```python
from build123d import *

# Parameters (mm, degrees)
F0_R     = 1.778
F0_W     = 19.05
F0_H     = 25.4
F0_R_2   = 1.7145
F1_DEPTH = 3.175
F2_DEPTH = 11.43


# Not quite as in the source:
# - a feature names something its author has since deleted; it is built from what else it names


with BuildPart() as f1:
    # F0 (on Top) → F1 (new body)
    with BuildSketch(Plane.XY):
        Polygon((-38.2503936946, 15.7646441165), (-38.2503936946, -9.6299967694), (139.5496063054, -9.6299967694), (139.5496063054, 15.7700032306), (12.5479004732, 15.7700032306), (-11.7069316009, 15.7700032306), (-38.2485270353, 15.7700032306), align=None)
        Polygon((20.5585099757, -3.2853558835), (20.5585099757, 3.0646441165), (20.5585099757, 9.4146441165), (25.6385099757, 9.4146441165), (25.6385099757, -3.2853558835), align=None, mode=Mode.SUBTRACT)
        Polygon((35.4481115937, -3.2853558835), (35.4481115937, 3.0646441165), (35.4481115937, 9.4146441165), (40.5281115937, 9.4146441165), (40.5281115937, -3.2853558835), align=None, mode=Mode.SUBTRACT)
        with Locations((50.6496063054, 3.0646441165)):
            Circle(F0_R, mode=Mode.SUBTRACT)
        with Locations((63.3496063054, 3.0646441165)):
            Circle(F0_R, mode=Mode.SUBTRACT)
        with Locations((76.0496063054, 3.0646441165)):
            Circle(F0_R, mode=Mode.SUBTRACT)
        with Locations((88.7496063054, 3.0646441165)):
            Circle(F0_R, mode=Mode.SUBTRACT)
        with Locations((101.4496063054, 3.0646441165)):
            Circle(F0_R, mode=Mode.SUBTRACT)
        with Locations((114.1496063054, 3.0646441165)):
            Circle(F0_R, mode=Mode.SUBTRACT)
        with Locations((126.8496063054, 3.0646441165)):
            Circle(F0_R, mode=Mode.SUBTRACT)
        Polygon((-44.6003936946, 15.7700032306), (-44.6003936946, -9.6299967694), (-38.2503936946, -9.6299967694), (-38.2503936946, 15.7646441165), (-38.2485270353, 15.7700032306), align=None)
        with Locations((-54.1253936946, 3.0700032306)):
            Rectangle(F0_W, F0_H)
        with Locations((-50.9503936946, 3.0646441165)):
            Circle(F0_R_2, mode=Mode.SUBTRACT)
        Polygon((-11.7069316009, 91.9700032306), (-38.2485270353, 15.7700032306), (-11.7069316009, 15.7700032306), align=None)
        Polygon((-11.7069316009, 91.9700032306), (-11.7069316009, 15.7700032306), (12.5479004732, 15.7700032306), align=None)
    extrude(amount=F1_DEPTH)

    # F0 (on Top) → F2 (join)
    with BuildSketch(Plane.XY):
        with Locations((-50.9503936946, 3.0646441165)):
            Circle(F0_R_2)
    extrude(amount=F2_DEPTH)


solid = f1.part
```
Could you check a few things on this model? Use its own coordinates, in mm. A direction names the side the tool comes from. Coordinates: 2 decimals unless noted, no trailing zeros. Loops run counter-clockwise (first coordinate to the right, second up) from the corner with the lowest first, then second, coordinate; pieces in that order, holes last. Notation, with made-up numbers: M 11,68.25 L 53,68.25 A28 ccw 53,105.25 Z; hole C 30.25,63 d4. An arc over 180 degrees is marked long. Put each result on its own line as item: value. Start each with the question number.
(1) Suppose I cut it at B-B on y = 13. Please give me the cut outline in (x, z) (3 decimals), then the cut area to 3 significant figures.
(2) Suppose I cut it at A-A on x = 23.5. Please give me the cut outline in (y, z) (3 decimals).
(3) Thinking about a two-plate mould opening in X: for faces 3 (the face through (115.846, 3.599, 1.565)), 4 (the face through (125.073, 3.143, 1.565)), 5 (the face through (0.6, 53.3, 1.6)), 6 (the face through (22, 11, 3.175)), which applies, pulls with the +X half, pulls with the -X half, needs draft (parallel to the pull), parting line crosses it, or undercut?
(4) Suppose I cut it at D-D on z = 8. Please give me the cut outline in (x, y), then the cut area to 3 significant figures.
(5) For faces 1 (the face through (-52.663, 3.14, 7.245)), 2 (the face through (90.446, 3.599, 1.565)), which set-ups out of +Z, -Z, +X, -X, +Y, -Y let a thin tool reach every point of the face, with its end or its side?
(6) Will these pins go through, and if not, where does the flat tip stop? P1, Ø1, axis at x = -52.5, z = 1.5, coming from the +Y side; P2, Ø5.5, axis at x = 126.85, y = 3.06, coming from the +Z side (3 decimals); P3, Ø3, axis at x = 114.15, y = 3.06, coming from the -Z side; P4, Ø3, axis at y = 75, z = 4, coming from the -X side.
(7) Suppose I cut it at C-C on x = 67.5. Please give me the cut outline in (y, z) (3 decimals).
(8) I need wall thicknesses on line 1 (Y direction, x = 24.5, z = 2.5); line 2 (Y direction, x = 72.5, z = 2.5); line 3 (Z direction, x = 84.5, y = 15) (3 decimals). Which ranges of each line are inside material? Lowest first, please. Write a range as from..to.
Solutions:
1. outline: M -63.65,0 L 139.55,0 L 139.55,3.175 L -63.65,3.175 Z
1. area: 645 mm2
2. outline: M -9.63,0 L -3.285,0 L -3.285,3.175 L -9.63,3.175 Z; M 9.415,0 L 15.77,0 L 15.77,3.175 L 9.415,3.175 Z
3. face 3: undercut
3. face 4: undercut
3. face 5: pulls with the +X half
3. face 6: needs draft
4. outline: C -50.95,3.06 d3.43
4. area: 9.23 mm2
5. face 1: +Z
5. face 2: +Z, -Z
6. P1: stops at y = 15.77
6. P2: stops at z = 3.175
6. P3: passes through
6. P4: stops at x = -18.05
7. outline: M -9.63,0 L 15.77,0 L 15.77,3.175 L -9.63,3.175 Z
8. line 1: y = -9.63..-3.29, 9.41..15.77
8. line 2: y = -9.63..15.77
8. line 3: z = 0..3.175
